The listing builds one solid part. Answer for the finished solid, in the listing's coordinates (mm). Give positions to 0.01 mm unless a question says otherwise; leave off trailing zeros.
```python
from build123d import *

# Parameters (mm, degrees)
F1_DEPTH = 3.175


# Not quite as in the source:
# - a length typed as a fraction of an inch, garbled in the dataset ("3 / 203.2 mm" for 3/8 in), is restored


with BuildPart() as f1:
    # F0 (on Top) → F1 (new body)
    with BuildSketch(Plane.XY):
        with BuildLine():
            Line((-67.493813857, 42.5679214677), (-92.893813857, 42.5679214677))
            Line((-92.893813857, 42.5679214677), (-92.893813857, -33.6320785323))
            add(Edge.make_bspline(
                [(-92.893813857, -33.6320785323), (-67.493813857, -53.2479426065), (-16.693813857, -64.816214458), (34.106186143, -53.2479426065), (59.506186143, -33.6320785323)],
                knots=[0, 0, 0, 0, 0.5, 1, 1, 1, 1], degree=3))
            Line((59.506186143, -33.6320785323), (59.506186143, 42.5679214677))
            Line((59.506186143, 42.5679214677), (34.106186143, 42.5679214677))
            Line((34.106186143, 42.5679214677), (8.706186143, 42.5679214677))
            ThreePointArc((8.706186143, 42.5679214677), (1.2666983851, 24.6074092256), (-16.693813857, 17.1679214677))
            ThreePointArc((-16.693813857, 17.1679214677), (-34.6543260992, 24.6074092256), (-42.093813857, 42.5679214677))
            Line((-42.093813857, 42.5679214677), (-67.493813857, 42.5679214677))
        make_face()
    extrude(amount=F1_DEPTH)


solid = f1.part
```
1) Straight lines are drawn through the part: probe 1 along X at (y, z) = (26, 1.65); probe 2 along X at (y, z) = (29, 3.05); probe 3 along X at (y, z) = (-34, 0.6). For each, find the intervals that lie inside material, in ascending order.
Geometry says:
probe 1: x = -92.89 to -35.95, 2.56 to 59.51
probe 2: x = -92.89 to -38.17, 4.78 to 59.51
probe 3: x = -92.42 to 59.03
2) Given P1, Ø2, axis at x = -75.5, y = 16.5, coming from the -Z side; P2, Ø1, axis at x = -28, z = 2.5, coming from the -Y side, each flat-ended and moving along its own axis, determine where each tip first touches the part or whether it passes through.
Geometry says:
P1: stops at z = 0
P2: stops at y = -58.66
3) For a pull along Z with two mould halves and no side action, classify faces 1 (the flat face through (-18, -10, 3.175)), 2 (the flat face through (-18, -10, 0)), 3 (the flat face through (34, 42.568, 2)) as +Z half, -Z half, draft (parallel to the pull), parting line (faces both ways), or undercut.
Geometry says:
face 1: +Z half
face 2: -Z half
face 3: draft
